The drawing under review shows one solid part. Ordinate dimensions are in mm from its lowest x, y, z. A direction names the side the tool comes from. Give positions to 0.01 mm unless a question says otherwise; leave off trailing zeros. Loops run counter-clockwise (first coordinate to the right, second up) from the corner with the lowest first, then second, coordinate; pieces in that order, holes last. Notation, with made-up numbers: M 32,60.25 L 90,60.25 A17 ccw 90,85.25 Z; hole C 20,57 d1. An arc over 180 degrees is marked long. Write item = value, one per line. Start each with the question number.
1. We need section B-B on x = 202. Give the boundary of the cut face in (y, z), then the cut area to 3 significant figures.
2. Wall thickness on line 1 along Z through (x, y) = (112.5, 25); line 2 along Y through (x, z) = (230, 26): over which ranges is each line inside the solid? List them lowest first. Write a range as from..to.
3. Draft analysis for pull direction Z (two halves, no side actions). For the marked faces 3, 4 and 5, state which applies: pulls with the +Z half, pulls with the -Z half, needs draft (parallel to the pull), parting line crosses it, or undercut.
4. For pin 1 (18 mm diameter, centred on x = 245, z = 40.5, fed in from -Y), flat-tipped, find the tip position at first contact; note if it passes through.
5. We need section C-C on z = 32. Give the boundary of the cut face in (x, y).
6. For the marked faces 1 and 2, list the 3-axis set-ups (+Z, -Z, +X, -X, +Y, -Y) from which the entire face can be reached by the end or side of a thin tool; tool diameter is ignored.
7. We need section A-A on y = 17.5. Give the boundary of the cut face in (x, z), then the cut area to 3 significant figures.
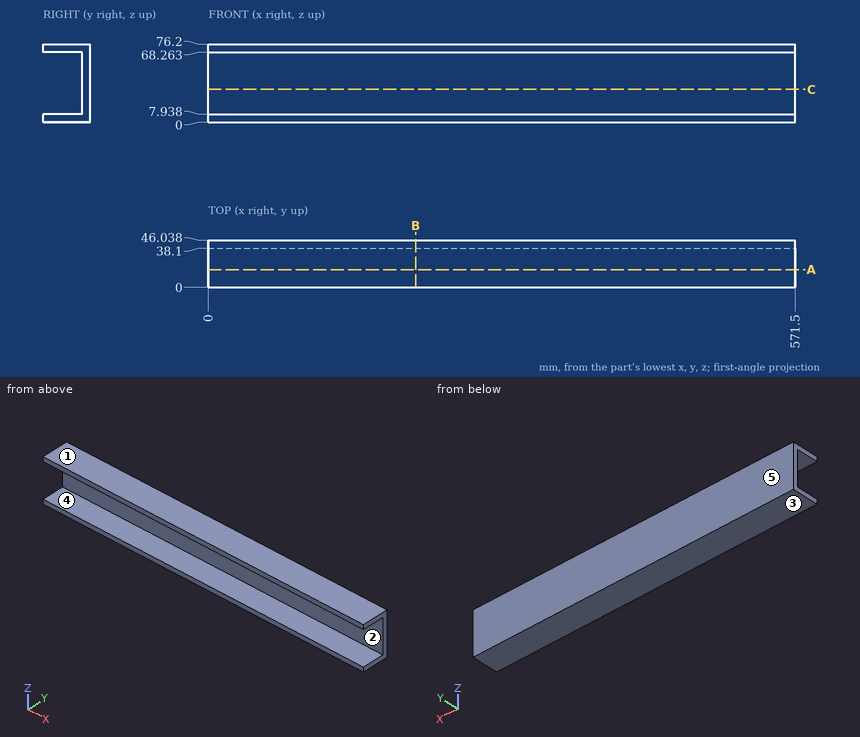
Final values:
q1.outline = M 0,0 L 46.04,0 L 46.04,76.2 L 0,76.2 L 0,68.26 L 38.1,68.26 L 38.1,7.94 L 0,7.94 Z
q1.area = 1,210 mm²
q2.line_1 = 0..7.94, 68.26..76.2
q2.line_2 = 38.1..46.04
q3.face_3 = pulls with the -Z half
q3.face_4 = undercut
q3.face_5 = needs draft
q4.pin_1 = 38.1
q5.outline = M 0,38.1 L 571.5,38.1 L 571.5,46.04 L 0,46.04 Z
q6.face_1 = +Z, +X, -X, +Y, -Y
q6.face_2 = +X, -X, -Y
q7.outline = M 0,0 L 571.5,0 L 571.5,7.94 L 0,7.94 Z; M 0,68.26 L 571.5,68.26 L 571.5,76.2 L 0,76.2 Z
q7.area = 9,070 mm²
